The listing builds one solid part. Answer for the finished solid, in the listing's coordinates (mm). A direction names the side the tool comes from. Give positions to 0.01 mm unless a question says otherwise; leave off trailing zeros. Order: outer loops, then holes, each group sorted by start corner. A loop starts at its lowest first (then second) coordinate and runs counter-clockwise, first axis right, second up. Notation, with made-up numbers: (4, 57.5) - (62, 57.5) arc R16 ccw to (62, 71.5) - close; hole circle Ø11 at (7.5, 68.5). An arc over 180 degrees is marked (long way). Write each question's results on one line, items separated by ' | '. Start each with the question number.
1. Section A-A (y = 0) is taken. Give the vertices of the cut face in (x, z).
2. Which of the six approach directions +Z, -Z, +X, -X, +Y, -Y give full straight-line access (tool end or side, diameter ignored) to faces 1 (the face through (1.845, 0, 18)), 2 (the face through (-2, -1, 15)), 3 (the face through (-6.155, 0, 17)), 4 (the face through (-4.655, 0, -10))?
3. Find the intervals of material crossed by L1, parallel to Y at x = 1.25, z = 37.5; L2, parallel to Z at x = -3.75, y = 0.25; L3, parallel to Z at x = -3, y = 2, in increasing order.
4. Section C-C (z = -6.5) is taken. Give the vertices of the cut face in (x, y), and give its area (3 significant figures).
5. Flat-ended cylindrical pins translate along their axes: pin 1 (2 mm diameter, centred on y = 0.5, z = 7, fed in from +X); pin 2 (2 mm diameter, centred on y = 2.5, z = 37.5, fed in from +X); pin 3 (2 mm diameter, centred on y = 0.5, z = 15.5, fed in from -X); pin 4 (3 mm diameter, centred on y = 4, z = 13.5, fed in from -X). Find the tip coordinate at first contact, or state that the pin passes through.
6. Section B-B (x = -2.75) is taken. Give the vertices of the cut face in (y, z).
7. Determine the mould class of faces 5 (the face through (-2, 6, 40)), 6 (the face through (0.345, 0, -10)), 7 (the face through (-3.113, 3.465, 42.765)) for opening direction Z: released by +Z, released by -Z, zero draft, split by the parting line, or undercut.
8. Section D-D (z = 32.5) is taken. Give the vertices of the cut face in (x, y).
from build123d import *

# Parameters (mm, degrees)
SKETCH1_W           = 5
SKETCH1_H           = 5
BOSS_EXTRUDE1_DEPTH = 1
FILLET1_R           = 1
SKETCH2_R           = 2.5
BOSS_EXTRUDE2_DEPTH = 5


with BuildPart() as part:
    # Sketch1 → Boss-Extrude1 (new, symmetric)
    # profile 1 of 2: a face of its own
    with BuildSketch(Plane(origin=(0, 0, 0), x_dir=(1, 0, 0), z_dir=(0, 1, 0))):
        with BuildLine():
            Line((1.844736842, 5.044736842), (-6.155263158, 5.044736842))
            Line((-6.155263158, 5.044736842), (-6.155263158, -40.455263158))
            ThreePointArc((-6.155263158, -40.455263158), (-2.155263158, -44.455263158), (1.844736842, -40.455263158))
            Line((1.844736842, -40.455263158), (1.844736842, 5.044736842))
        make_face()
    # profile 2 of 2: a face of its own
    with BuildSketch(Plane(origin=(0, 0, 0), x_dir=(1, 0, 0), z_dir=(0, 1, 0))):
        Polygon((-6.655263158, 5.044736842), (-6.155263158, 5.044736842), (1.844736842, 5.044736842), (2.344736842, 5.044736842), (2.344736842, 14.044736842), (-6.655263158, 14.044736842), align=None)
        with Locations((-2.155263158, 9.544736842)):
            Rectangle(SKETCH1_W, SKETCH1_H, mode=Mode.SUBTRACT)
    extrude(amount=BOSS_EXTRUDE1_DEPTH, both=True)

    # Fillet1
    # the kernel refuses this fillet: 1 mm, written as the material it takes off along each edge
    with BuildSketch(Plane(origin=(2.344736842, 3.165063509, -5.044736842), x_dir=(0, 0, -1), z_dir=(0, -1, 0)), Plane(origin=(-6.655263158, -3.165063509, -5.044736842), x_dir=(0, 0, -1), z_dir=(0, 1, 0))) as fillet1_piece_1:
        with BuildLine():
            CenterArc((0.866025404, -1), FILLET1_R, 90, 60)
            Line((0, -0.5), (-0.017320508, -0.49))
            ThreePointArc((-0.017320508, -0.49), (-0.02, -0.25), (-0.02, 0))
            Line((-0.02, 0), (0, 0.02))
            Line((0, 0.02), (0.866025404, 0.02))
            Line((0.866025404, 0.02), (0.866025404, 0))
        make_face()
    extrude(amount=6.330127019, mode=Mode.SUBTRACT)
    with BuildSketch(Plane(origin=(2.344736842, 3.5, -14.044736842), x_dir=(-1, 0, 0), z_dir=(0, -1, 0)), Plane(origin=(-6.655263158, -3.5, -14.044736842), x_dir=(1, 0, 0), z_dir=(0, 1, 0))) as fillet1_piece_2:
        with BuildLine():
            CenterArc((FILLET1_R, -FILLET1_R), FILLET1_R, 90, 90)
            Line((0, -FILLET1_R), (-FILLET1_R * 0.02, -FILLET1_R))
            Line((-FILLET1_R * 0.02, -FILLET1_R), (-FILLET1_R * 0.02, FILLET1_R * 0.02))
            Line((-FILLET1_R * 0.02, FILLET1_R * 0.02), (FILLET1_R, FILLET1_R * 0.02))
            Line((FILLET1_R, FILLET1_R * 0.02), (FILLET1_R, 0))
        make_face()
    extrude(amount=7, mode=Mode.SUBTRACT)

    # Sketch2 → Boss-Extrude2 (add)
    with BuildSketch(Plane(origin=(0, 1, 0), x_dir=(1, 0, 0), z_dir=(0, 1, 0))):
        with Locations(Location((-2.155263158, -40.455263158, 0), (0, 0, 270))):
            Circle(SKETCH2_R)
    extrude(amount=BOSS_EXTRUDE2_DEPTH)


solid = part.part
Reported:
1) outline: (-6.66, -13.04) arc R1 ccw to (-5.66, -14.04) - (1.34, -14.04) arc R1 ccw to (2.34, -13.04) - (2.34, -5.91) arc R1 ccw to (1.84, -5.04) - (1.84, 40.46) arc R4 ccw to (-6.16, 40.46) - (-6.16, -5.04) arc R1 ccw to (-6.66, -5.91) - close; hole (-4.66, -12.04) - (0.34, -12.04) - (0.34, -7.04) - (-4.66, -7.04) - close
2) face 1: +Z, +X, +Y, -Y | face 2: +Z, -Z, +X, -X, -Y | face 3: +Z, -X, +Y, -Y | face 4: +Y, -Y
3) L1: -1 to 1 | L2: -14.04 to -12.04, -7.04 to 44.12 | L3: 38.1 to 42.81
4) outline: (-6.66, -1) - (2.34, -1) - (2.34, 1) - (-6.66, 1) - close | area: 18.0 mm²
5) pin 1: x = 1.84 | pin 2: x = -0.6 | pin 3: x = -6.16 | pin 4: through
6) outline: (-1, -14.04) - (1, -14.04) - (1, -12.04) - (-1, -12.04) - close; (-1, -7.04) - (1, -7.04) - (1, 38.03) - (6, 38.03) - (6, 42.88) - (1, 42.88) - (1, 44.41) - (-1, 44.41) - close
7) face 5: zero draft | face 6: undercut | face 7: split by the parting line
8) outline: (-6.16, -1) - (1.84, -1) - (1.84, 1) - (-6.16, 1) - close
